The model under review builds one solid part; all positions refer to its coordinate system, in mm. A direction names the side the tool comes from. Coordinates: 2 decimals unless noted, no trailing zeros. Loops run counter-clockwise (first coordinate to the right, second up) from the corner with the lowest first, then second, coordinate; pieces in that order, holes last. Notation, with made-up numbers: (40.5, -30.75) - (51.5, -30.75) arc R18 cw to (51.5, -4.75) - close; hole circle Ø3 at (44.5, 51.5). An arc over 180 degrees is marked (long way). One line per item, written item: value. Start each with the question number.
1. We need section B-B, the plane x = 7.5. Give the boundary of the cut face in (y, z).
2. Insertion check: P1, Ø4, axis at x = 2.5, z = 2.5, coming from the -Y side; P2, Ø0.6, axis at y = 0.5, z = 13.5, coming from the -X side; P3, Ø0.5, axis at x = 5, y = 2, coming from the -Z side; P4, Ø0.6, axis at x = -3, z = 14.5, coming from the -Y side. Each pin has a flat end and moves straight along its axis. Give the tip position at first contact, or say it passes through.
3. For faces 1 (the face through (-9.5, 1, 15)), 2 (the face through (0, -2.5, 3)), 3 (the face through (0, -3, 12)), 4 (the face through (-3, 2.5, 7)), 5 (the face through (9.199, -2.215, 11.014)), list the 3-axis set-ups (+Z, -Z, +X, -X, +Y, -Y) from which the entire face can be reached by the end or side of a thin tool; tool diameter is ignored.
4. To check wall thickness, follow line 1 (X direction, y = 1, z = 6.5); line 2 (Z direction, x = -7.5, y = -3); line 3 (Y direction, x = -4.5, z = 2.75). State the ranges of each line that lie inside material, in increasing order.
5. We need section D-D, the plane y = -0.25. Count the separate pieces of the cut face and the enclosed holes in it, then the cut area to 3 significant figures.
6. Mouldability with a two-part tool opening along Y and no side actions: class faces 6 (the face through (-10.215, -3.199, 1.014)), 7 (the face through (3, 2.498, 16)), 8 (the face through (9.5, 1, 15)), 9 (the face through (0, 3.5, 9)) as +Y half, -Y half, draft (parallel to the pull), parting line (faces both ways), or undercut.
from build123d import *

# Parameters (mm, degrees)
SKETCH2_W            = 21
SKETCH2_H            = 7
BOSS_EXTRUDE1_DEPTH  = 2
SKETCH3_W            = 19
SKETCH3_H            = 6
BOSS_EXTRUDE2_DEPTH  = 2
SKETCH4_W            = 21
SKETCH4_H            = 7
BOSS_EXTRUDE3_DEPTH  = 2
SKETCH5_W            = 19
SKETCH5_H            = 6
BOSS_EXTRUDE4_DEPTH  = 2
SKETCH6_W            = 21
SKETCH6_H            = 7
BOSS_EXTRUDE5_DEPTH  = 2
SKETCH7_W            = 19
SKETCH7_H            = 6
BOSS_EXTRUDE6_DEPTH  = 2
SKETCH8_W            = 21
SKETCH8_H            = 7
BOSS_EXTRUDE7_DEPTH  = 2
FILLET1_R            = 1
CUT_EXTRUDE2_DEPTH   = 14
SKETCH13_W           = 2.12863245
SKETCH13_H           = 3.140125133
BOSS_EXTRUDE9_DEPTH  = 14
SKETCH14_W           = 19
SKETCH14_H           = 6
BOSS_EXTRUDE10_DEPTH = 2
SKETCH15_W           = 21.003804152
SKETCH15_H           = 7.001896417
BOSS_EXTRUDE11_DEPTH = 2
FILLET2_R            = 1
CUT_EXTRUDE4_DEPTH   = 4
SKETCH17_W           = 2.12863245
SKETCH17_H           = 2.998103583
BOSS_EXTRUDE12_DEPTH = 4


with BuildPart() as part:
    # Sketch2 → Boss-Extrude1 (new body)
    with BuildSketch(Plane.XY):
        Rectangle(SKETCH2_W, SKETCH2_H)
    extrude(amount=BOSS_EXTRUDE1_DEPTH)

    # Sketch3 → Boss-Extrude2 (add)
    with BuildSketch(Plane.XY.offset(2)):
        with Locations((0, 0.5)):
            Rectangle(SKETCH3_W, SKETCH3_H)
    extrude(amount=BOSS_EXTRUDE2_DEPTH)

    # Sketch4 → Boss-Extrude3 (add)
    with BuildSketch(Plane.XY.offset(4)):
        Rectangle(SKETCH4_W, SKETCH4_H)
    extrude(amount=BOSS_EXTRUDE3_DEPTH)

    # Sketch5 → Boss-Extrude4 (add)
    with BuildSketch(Plane.XY.offset(6)):
        with Locations((0, 0.5)):
            Rectangle(SKETCH5_W, SKETCH5_H)
    extrude(amount=BOSS_EXTRUDE4_DEPTH)

    # Sketch6 → Boss-Extrude5 (add)
    with BuildSketch(Plane.XY.offset(8)):
        Rectangle(SKETCH6_W, SKETCH6_H)
    extrude(amount=BOSS_EXTRUDE5_DEPTH)

    # Sketch7 → Boss-Extrude6 (add)
    with BuildSketch(Plane.XY.offset(10)):
        with Locations((0, 0.5)):
            Rectangle(SKETCH7_W, SKETCH7_H)
    extrude(amount=BOSS_EXTRUDE6_DEPTH)

    # Sketch8 → Boss-Extrude7 (add)
    with BuildSketch(Plane.XY.offset(12)):
        Rectangle(SKETCH8_W, SKETCH8_H)
    extrude(amount=BOSS_EXTRUDE7_DEPTH)

    # Fillet1
    fillet1_edges = [part.edges().sort_by_distance(p)[0] for p in [
        (-9.5, -2.5, 3),
        (9.5, -2.5, 3),
        (-10.5, -3.5, 5),
        (10.5, -3.5, 5),
        (-9.5, -2.5, 7),
        (9.5, -2.5, 7),
        (10.5, -3.5, 9),
        (-10.5, -3.5, 9),
        (-9.5, -2.5, 11),
        (9.5, -2.5, 11),
        (10.5, -3.5, 1),
        (-10.5, -3.5, 13),
        (10.5, -3.5, 13),
        (-10.5, -3.5, 1),
    ]]
    fillet(fillet1_edges, radius=FILLET1_R)

    # Sketch12 → Cut-Extrude2 (cut)
    with BuildSketch(Plane(origin=(0, 0, 0), x_dir=(-1, 0, 0), z_dir=(0, 0, -1))):
        with BuildLine():
            Line((-5.5, 2.5), (5.5, 2.5))
            ThreePointArc((5.5, 2.5), (7, 1), (5.5, -0.5))
            Line((5.5, -0.5), (-5.5, -0.5))
            ThreePointArc((-5.5, -0.5), (-7, 1), (-5.5, 2.5))
        make_face()
    extrude(amount=-CUT_EXTRUDE2_DEPTH, mode=Mode.SUBTRACT)

    # Sketch13 → Boss-Extrude9 (add)
    with BuildSketch(Plane(origin=(0, 0, 0), x_dir=(-1, 0, 0), z_dir=(0, 0, -1))):
        with Locations((0, 1.070062567)):
            Rectangle(SKETCH13_W, SKETCH13_H)
    extrude(amount=-BOSS_EXTRUDE9_DEPTH)

    # Sketch14 → Boss-Extrude10 (add)
    with BuildSketch(Plane.XY.offset(14)):
        with Locations((0, 0.5)):
            Rectangle(SKETCH14_W, SKETCH14_H)
    extrude(amount=BOSS_EXTRUDE10_DEPTH)

    # Sketch15 → Boss-Extrude11 (add)
    with BuildSketch(Plane.XY.offset(16)):
        with Locations((-0.001902076, -0.000948209)):
            Rectangle(SKETCH15_W, SKETCH15_H)
    extrude(amount=BOSS_EXTRUDE11_DEPTH)

    # Fillet2
    fillet2_edges = [part.edges().sort_by_distance(p)[0] for p in [
        (9.5, -2.5, 15),
        (-9.5, -2.5, 15),
        (10.5, -3.501896417, 17),
        (-10.503804152, -3.501896417, 17),
    ]]
    fillet(fillet2_edges, radius=FILLET2_R)

    # Sketch16 → Cut-Extrude4 (cut)
    with BuildSketch(Plane.XY.offset(18)):
        with BuildLine():
            Line((5.5, -0.501896417), (-5.5, -0.501896417))
            ThreePointArc((-5.5, -0.501896417), (-7, 0.998103583), (-5.5, 2.498103583))
            Line((-5.5, 2.498103583), (5.5, 2.498103583))
            ThreePointArc((5.5, 2.498103583), (7, 0.998103583), (5.5, -0.501896417))
        make_face()
    extrude(amount=-CUT_EXTRUDE4_DEPTH, mode=Mode.SUBTRACT)

    # Sketch17 → Boss-Extrude12 (add)
    with BuildSketch(Plane.XY.offset(18)):
        with Locations((0, 0.999051792)):
            Rectangle(SKETCH17_W, SKETCH17_H)
    extrude(amount=-BOSS_EXTRUDE12_DEPTH)


solid = part.part
Findings below:
1. outline: (-3.5, 0) - (3.5, 0) - (3.5, 18) - (-3.5, 18) - (-3.5, 16) - (-2.5, 16) - (-2.5, 14) - (-3.5, 14) - (-3.5, 12) - (-2.5, 12) - (-2.5, 10) - (-3.5, 10) - (-3.5, 8) - (-2.5, 8) - (-2.5, 6) - (-3.5, 6) - (-3.5, 4) - (-2.5, 4) - (-2.5, 2) - (-3.5, 2) - close
2. P1: y = -3.5
2. P2: x = -10.5
2. P3: through
2. P4: y = -2.5
3. face 1: -X, +Y, -Y
3. face 2: +X, -X, -Y
3. face 3: -Y
3. face 4: +Z, -Z
3. face 5: +X, -Y
4. line 1: -9.5 to -7, -1.06 to 1.06, 7 to 9.5
4. line 2: 0 to 2, 4 to 6, 8 to 10, 12 to 14, 16 to 18
4. line 3: -2.5 to -0.5, 2.5 to 3.5
5. separate pieces: 3
5. enclosed holes: 0
5. area: 172 mm2
6. face 6: -Y half
6. face 7: undercut
6. face 8: draft
6. face 9: +Y half
